Here's how the part is built. I have some questions about the finished solid (model axes, mm). A direction names the side the tool comes from. Coordinates: 2 decimals unless noted, no trailing zeros. Use one line per item in the form item = value. Start each with the question number.
(1) On a 3-axis mill with a long thin cutter (end or side, diameter ignored), from which of +Z, -Z, +X, -X, +Y, -Y can I reach the whole of each face in a straight line? I mean faces 1 (the flat face through (133, 0, 20)), 2 (the cylindrical face through (5.9, 22.4, 18.2)), 3 (the cylindrical face through (264.1, 17.6, 18.2)). Say none if no direction works.
(2) Please list where this line runs through material, in increasing order: L1, parallel to Z at x = 261.25, y = 20.
(3) Will these pins go through, and if not, where does the flat tip stop? P1, Ø6.5, axis at y = 21.5, z = 21, coming from the -X side; P2, Ø1.8, axis at y = 20, z = 21.5, coming from the +X side.
(4) Thinking about a two-plate mould opening in Y: for faces 4 (the flat face through (133, 20, 0)), 5 (the flat face through (133, 40, 20)), 6 (the flat face through (12, 20, 20)), which applies, +Y half, -Y half, draft (parallel to the pull), parting line (faces both ways), or undercut?
```python
from build123d import *

# Parameters (mm, degrees)
F0_W     = 40
F0_H     = 40
F1_DEPTH = 270
F2_R     = 3
F3_DEPTH = 12
F4_R     = 3
F5_DEPTH = 12


with BuildPart() as f1:
    # F0 (on Right) → F1 (new body)
    with BuildSketch(Plane.YZ):
        with Locations((20, 20)):
            Rectangle(F0_W, F0_H)
    extrude(amount=F1_DEPTH)

    # F2 (on face) → F3 (cut)
    with BuildSketch(Plane.YZ.offset(270)):
        with Locations((20, 20)):
            Circle(F2_R)
    extrude(amount=-F3_DEPTH, mode=Mode.SUBTRACT)

    # F4 (on face) → F5 (cut)
    with BuildSketch(Plane(origin=(0, 0, 0), x_dir=(0, -1, 0), z_dir=(-1, 0, 0))):
        with Locations((-20, 20)):
            Circle(F4_R)
    extrude(amount=-F5_DEPTH, mode=Mode.SUBTRACT)


solid = f1.part
```
Answer:
q1.face_1 = +Z, -Z, +X, -X, -Y
q1.face_2 = -X
q1.face_3 = +X
q2.L1 = 0 to 17, 23 to 40
q3.P1 = 0
q3.P2 = 258
q4.face_4 = draft
q4.face_5 = +Y half
q4.face_6 = undercut
